Autodesk Inventor part; units mm, degrees
ref_plane "YZ Plane" through (0, 0, 0) normal (1, 0, 0) x (0, 1, 0)
ref_plane "XZ Plane" through (0, 0, 0) normal (0, 1, 0) x (-1, 0, 0)
ref_plane "XY Plane" through (0, 0, 0) normal (0, 0, 1) x (1, 0, 0)
sketch "Sketch1" plane through (0, 0, 0) normal (0, 0, 1) x (1, 0, 0)
  line L0 (0, 0) -> (1684, 0)
  line L1 (1684, 0) -> (1684, 955)
  line L2 (1684, 955) -> (0, 955)
  line L3 (0, 955) -> (0, 0)
  dimension "d0" = 1684
  dimension "d1" = 955
extrude "Extrusion1" add sketch "Sketch1" along normal blind 61
fillet "Fillet1" radius 10 4 edges at (0, 477.5, 0) (842, 955, 0) (842, 0, 0) (1684, 477.5, 0)
sketch "Sketch2" plane through (0, 0, 0) normal (0, 0, -1) x (-1, 0, 0)
  point P0 (0, 0)
sketch "Sketch3" plane through (0, 0, 0) normal (0, 0, -1) x (-1, 0, 0)
  line L0 (-1658.1713, 929.1713) -> (-29.133, 929.1713)
  line L1 (-29.133, 929.1713) -> (-29.133, 29.4852)
  line L2 (-29.133, 29.4852) -> (-1658.1713, 29.4852)
  line L3 (-1658.1713, 29.4852) -> (-1658.1713, 929.1713)
  point P0 (0, 0)
extrude "Extrusion2" cut sketch "Sketch3" against normal blind 5
properties part number "TV"
CAD build for the part. Positions are in the model's coordinates, mm. Coordinates: 2 decimals unless noted, no trailing zeros. Order: outer loops, then holes, each group sorted by start corner. A loop starts at its lowest first (then second) coordinate and runs counter-clockwise, first axis right, second up. Notation, with made-up numbers: M 25,-24 L 65,-24 A21 ccw 65,5 Z; hole C -12,88.25 d4. An arc over 180 degrees is marked long. Write each question's results on one line, items separated by ' | '. Start each with the question number.
Q1. Flat gauge pins, fed straight in: P1, Ø5.5, axis at x = 719.5, z = 2, coming from the +Y side; P2, Ø3, axis at y = 574.5, z = 7.5, coming from the +X side; P3, Ø2, axis at x = 1095, y = 346, coming from the -Z side; P4, Ø6, axis at x = 981, z = 27, coming from the -Y side. Where does each tip first touch, or does it go through?
Q2. Drill centre lines: probe 1 along Z at (x, y) = (378.5, 820); probe 2 along Y at (x, z) = (1027, 9); probe 3 along X at (y, z) = (211, 6.5). Where is each one in solid material? Low to high. Write a range as from..to.
Q3. Pull direction X, two halves, no side cores. Call faces 1 (the flat face through (830, 0, 35)), 2 (the flat face through (0, 484, 35)), 3 (the flat face through (1684, 471, 35)), 4 (the flat face through (855, 486, 5)): +X half, -X half, draft (parallel to the pull), parting line (faces both ways), or undercut.
Q4. Cut at A-A (x = 432.5). List the corners of the cut face in (y, z), then the cut area to 3 significant figures.
Q5. Cut at B-B (y = 765.5). List the corners of the cut face in (x, z).
Found:
1) P1: y = 953.51 | P2: x = 1683.95 | P3: z = 5 | P4: y = 0
2) probe 1: 5..61 | probe 2: 0.05..954.95 | probe 3: 0.63..1683.37
3) face 1: draft | face 2: -X half | face 3: +X half | face 4: undercut
4) outline: M 0,10 A10 ccw 10,0 L 29.49,0 L 29.49,5 L 929.17,5 L 929.17,0 L 945,0 A10 ccw 955,10 L 955,61 L 0,61 Z | area: 53,700 mm²
5) outline: M 0,10 A10 ccw 10,0 L 29.13,0 L 29.13,5 L 1658.17,5 L 1658.17,0 L 1674,0 A10 ccw 1684,10 L 1684,61 L 0,61 Z
